Autodesk Inventor part; units mm, degrees
ref_plane "YZ Plane" through (0, 0, 0) normal (1, 0, 0) x (0, 1, 0)
ref_plane "XZ Plane" through (0, 0, 0) normal (0, 1, 0) x (-1, 0, 0)
ref_plane "XY Plane" through (0, 0, 0) normal (0, 0, 1) x (1, 0, 0)
sketch "Sketch1" plane through (0, 0, 0) normal (0, 0, 1) x (1, 0, 0)
  line L0 (-10.4542, 14.6019) -> (210.2083, 14.6019)
  line L1 (216.5583, 8.2519) -> (216.5583, -98.1106)
  line L2 (210.2083, -104.4606) -> (-10.4542, -104.4606)
  line L3 (-16.8042, -98.1106) -> (-16.8042, 8.2519)
  line L4 (99.877, 12.2207) -> (-10.4542, 12.2207)
  line L5 (-14.423, 8.2519) -> (-14.423, -44.9293)
  line L6 (99.877, 12.2207) -> (210.2083, 12.2207)
  line L7 (214.177, 8.2519) -> (214.177, -44.9293)
  line L8 (99.877, -102.0793) -> (210.2083, -102.0793)
  line L9 (214.177, -98.1106) -> (214.177, -44.9293)
  line L10 (99.877, -102.0793) -> (-10.4542, -102.0793)
  line L11 (-14.423, -98.1106) -> (-14.423, -44.9293)
  arc A0 (-10.4542, 14.6019) -> (-16.8042, 8.2519) centre (-10.4542, 8.2519) ccw
  arc A1 (216.5583, 8.2519) -> (210.2083, 14.6019) centre (210.2083, 8.2519) ccw
  arc A2 (210.2083, -104.4606) -> (216.5583, -98.1106) centre (210.2083, -98.1106) ccw
  arc A3 (-16.8042, -98.1106) -> (-10.4542, -104.4606) centre (-10.4542, -98.1106) ccw
  arc A4 (-10.4542, 12.2207) -> (-14.423, 8.2519) centre (-10.4542, 8.2519) ccw
  arc A5 (214.177, 8.2519) -> (210.2083, 12.2207) centre (210.2083, 8.2519) ccw
  arc A6 (210.2083, -102.0793) -> (214.177, -98.1106) centre (210.2083, -98.1106) ccw
  arc A7 (-14.423, -98.1106) -> (-10.4542, -102.0793) centre (-10.4542, -98.1106) ccw
  line L12 (99.877, 2.6957) -> (22.0895, 2.6957)
  line L13 (22.0895, 2.6957) -> (22.0895, -44.9293)
  line L14 (99.877, 2.6957) -> (182.427, 2.6957)
  line L15 (182.427, 2.6957) -> (182.427, -44.9293)
  line L16 (99.877, -92.5543) -> (182.427, -92.5543)
  line L17 (182.427, -92.5543) -> (182.427, -44.9293)
  line L18 (99.877, -92.5543) -> (22.0895, -92.5543)
  line L19 (22.0895, -92.5543) -> (22.0895, -44.9293)
  point P0 (0, 0)
  point P1 (-16.8042, 14.6019)
  point P2 (216.5583, -104.4606)
  point P3 (216.5583, 14.6019)
  point P4 (-16.8042, -104.4606)
  dimension "d0" = 233.3625
  dimension "d1" = 119.0625
  dimension "d9" = 6.35
  dimension "d10" = 3.9688
  dimension "d37" = 31.75
  dimension "d38" = 36.5125
  dimension "d39" = 9.525
  dimension "d40" = 9.525
extrude "Extrusion5" add sketch "Sketch1" along normal blind 2.3813 contours L0 A1 L1 A2 L2 A3 L3 A0 | L6 A5 L7 L9 A6 L8 L10 A7 L11 L5 A4 L4
sketch "Sketch6" plane through (0, 0, 2.3813) normal (0, 0, 1) x (1, 0, 0)
  line L0 (210.2083, 14.6019) -> (-10.4542, 14.6019)
  arc A0 (-10.4542, 14.6019) -> (-16.8042, 8.2519) centre (-10.4542, 8.2519) ccw
  line L1 (-16.8042, 8.2519) -> (-16.8042, -98.1106)
  arc A1 (-16.8042, -98.1106) -> (-10.4542, -104.4606) centre (-10.4542, -98.1106) ccw
  line L2 (-10.4542, -104.4606) -> (210.2083, -104.4606)
  arc A2 (210.2083, -104.4606) -> (216.5583, -98.1106) centre (210.2083, -98.1106) ccw
  line L3 (216.5583, -98.1106) -> (216.5583, 8.2519)
  arc A3 (216.5583, 8.2519) -> (210.2083, 14.6019) centre (210.2083, 8.2519) ccw
  line L4 (99.877, 12.2207) -> (-10.4542, 12.2207)
  line L5 (-14.423, 8.2519) -> (-14.423, -44.9293)
  line L6 (99.877, 12.2207) -> (210.2083, 12.2207)
  line L7 (214.177, 8.2519) -> (214.177, -44.9293)
  line L8 (99.877, -102.0793) -> (210.2083, -102.0793)
  line L9 (214.177, -98.1106) -> (214.177, -44.9293)
  line L10 (99.877, -102.0793) -> (-10.4542, -102.0793)
  line L11 (-14.423, -98.1106) -> (-14.423, -44.9293)
  arc A4 (-10.4542, 12.2207) -> (-14.423, 8.2519) centre (-10.4542, 8.2519) ccw
  arc A5 (214.177, 8.2519) -> (210.2083, 12.2207) centre (210.2083, 8.2519) ccw
  arc A6 (210.2083, -102.0793) -> (214.177, -98.1106) centre (210.2083, -98.1106) ccw
  arc A7 (-14.423, -98.1106) -> (-10.4542, -102.0793) centre (-10.4542, -98.1106) ccw
  point P0 (0, 0)
  dimension "d47" = 3.9688
extrude "Extrusion6" add sketch "Sketch6" along normal blind 2.3813
sketch "Sketch12" plane through (0, 0, 0) normal (0, 0, -1) x (-1, 0, 0)
  arc A0 (-210.2083, 14.6019) -> (-216.5583, 8.2519) centre (-210.2083, 8.2519) ccw
  arc A1 (-216.5583, -98.1106) -> (-210.2083, -104.4606) centre (-210.2083, -98.1106) ccw
  arc A2 (10.4542, -104.4606) -> (16.8042, -98.1106) centre (10.4542, -98.1106) ccw
  arc A3 (16.8042, 8.2519) -> (10.4542, 14.6019) centre (10.4542, 8.2519) ccw
  point P0 (0, 0)
hole "Hole2" at (210.2083, 8.2519, 0) at (-10.4542, 8.2519, 0) at (-10.4542, -98.1106, 0) at (210.2083, -98.1106, 0) direction (0, 0, 1) diameter 3.175 end through all
properties part number "Master Tablet Cover"
Input: part model. Units: mm. Frame: model coordinates. A direction names the side the tool comes from. Give positions to 0.01 mm unless a question says otherwise; leave off trailing zeros. Order: outer loops, then holes, each group sorted by start corner. A loop starts at its lowest first (then second) coordinate and runs counter-clockwise, first axis right, second up.
1. Set-up query: faces 1 (the face through (73, 7, 2.381)), 2 (the face through (-16.804, -44, 2)). Return all of +Z, -Z, +X, -X, +Y, -Y with unobstructed straight access to the full face (end or side cutting, diameter ignored); none if empty.
Computed:
face 1: +Z
face 2: +Z, -Z, -X, +Y, -Y
2. Cut plane A-A (z = 3.8). Return loops of the section in (x, y).
Computed:
outline: (-16.8, -98.11) arc R6.35 ccw to (-10.45, -104.46) - (210.21, -104.46) arc R6.35 ccw to (216.56, -98.11) - (216.56, 8.25) arc R6.35 ccw to (210.21, 14.6) - (-10.45, 14.6) arc R6.35 ccw to (-16.8, 8.25) - close; hole (-14.42, -98.11) arc R3.97 ccw to (-10.45, -102.08) - (210.21, -102.08) arc R3.97 ccw to (214.18, -98.11) - (214.18, 8.25) arc R3.97 ccw to (210.21, 12.22) - (-10.45, 12.22) arc R3.97 ccw to (-14.42, 8.25) - close
3. Pin query (flat end, axial travel): pin 1 Ø3 at (x, y) = (-10.45, -98.11) entering from +Z; pin 2 Ø5 at (x, y) = (210.21, 8.25) entering from -Z. Return the tip coordinate at first contact, or that it passes through.
Computed:
pin 1: passes through
pin 2: stops at z = 0
4. Cut plane C-C (y = -59). Return loops of the section in (x, z).
Computed:
outline: (-16.8, 0) - (22.09, 0) - (22.09, 2.38) - (-14.42, 2.38) - (-14.42, 4.76) - (-16.8, 4.76) - close; (182.43, 0) - (216.56, 0) - (216.56, 4.76) - (214.18, 4.76) - (214.18, 2.38) - (182.43, 2.38) - close
5. Draft query along X for faces 3 (the face through (99, 13, 4.763)), 4 (the face through (-13.29, 11.03, 3.56)), 5 (the face through (214.7, -102.6, 2.3)), 6 (the face through (212.98, 11.09, 3.56)). Return one class per face: released by +X, released by -X, zero draft, split by the parting line, or undercut.
Computed:
face 3: zero draft
face 4: undercut
face 5: released by +X
face 6: undercut
6. Line query: probe 1 along X at (y, z) = (-86, 3.5); probe 2 along Y at (x, z) = (48.5, 4.4); probe 3 along X at (y, z) = (-18, 1.65). Output: solid intervals per line, ascending.
Computed:
probe 1: x = -16.8 to -14.42, 214.18 to 216.56
probe 2: y = -104.46 to -102.08, 12.22 to 14.6
probe 3: x = -16.8 to 22.09, 182.43 to 216.56
7. Cut plane D-D (x = 202). Return loops of the section in (y, z), and give its area (3 significant figures).
Computed:
outline: (-104.46, 0) - (14.6, 0) - (14.6, 4.76) - (12.22, 4.76) - (12.22, 2.38) - (-102.08, 2.38) - (-102.08, 4.76) - (-104.46, 4.76) - close
area: 295 mm2
8. Cut plane B-B (x = 132). Return loops of the section in (y, z).
Computed:
outline: (-104.46, 0) - (-92.55, 0) - (-92.55, 2.38) - (-102.08, 2.38) - (-102.08, 4.76) - (-104.46, 4.76) - close; (2.7, 0) - (14.6, 0) - (14.6, 4.76) - (12.22, 4.76) - (12.22, 2.38) - (2.7, 2.38) - close
